Design review of the part shown in the three views and the two pictorial views. Dimensions are in mm from the part's minimum x, y and z. A direction names the side the tool comes from. Round coordinates to 2 decimals unless told otherwise and drop trailing zeros. Order: outer loops, then holes, each group sorted by start corner. A loop starts at its lowest first (then second) coordinate and runs counter-clockwise, first axis right, second up.
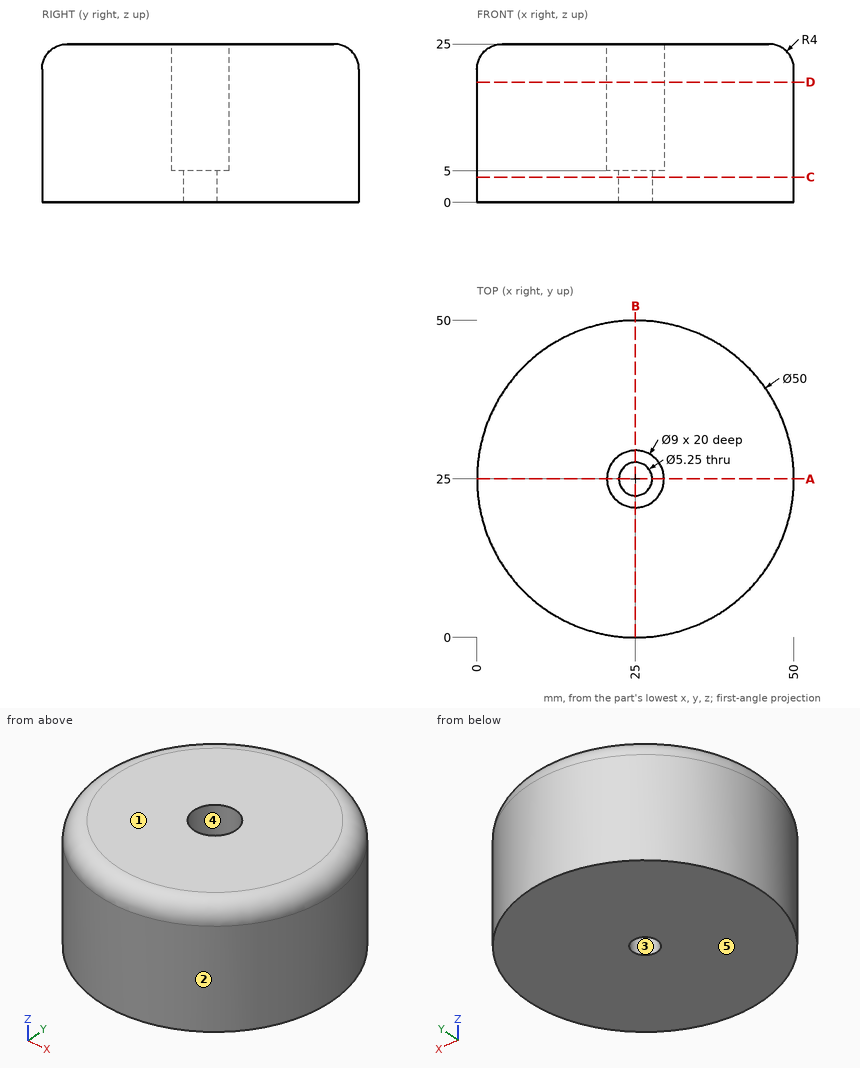
(1) Clearance check with flat-ended pins moving along their axes: P1, Ø1, axis at y = 32, z = 7.5, coming from the -X side; P2, Ø5, axis at y = 5, z = 12, coming from the -X side; P3, Ø11.5, axis at x = 25, y = 25, coming from the +Z side; P4, Ø4.5, axis at x = 24, y = 25, coming from the +Z side. State where each tip first meets the part, or that it passes through.
(2) Add section A-A on y = 25. Give the boundary of the cut face in (x, z) (3 decimals).
(3) Tool access review of the marked faces 4 and 5: name each direction out of +Z, -Z, +X, -X, +Y, -Y from which nothing blocks a thin tool from reaching the whole face with its end or side.
(4) Wall thickness on L1, parallel to Y at x = 25, z = 17.75; L2, parallel to Y at x = 25, z = 1.6 (3 decimals); L3, parallel to Y at x = 3, z = 7.25: over which ranges is each line inside the solid? List them lowest first.
(5) Add section D-D on z = 19. Give the boundary of the cut face in (x, y).
(6) Draft analysis for pull direction Y (two halves, no side actions). For the marked faces 1, 2 and 3, state which applies: pulls with the +Y half, pulls with the -Y half, needs draft (parallel to the pull), parting line crosses it, or undercut.
(7) Add section C-C on z = 4. Give the boundary of the cut face in (x, y) (3 decimals), plus the area to 3 significant figures.
Here are the results:
1. P1: stops at x = 0.86
1. P2: stops at x = 7.15
1. P3: stops at z = 25
1. P4: stops at z = 5
2. outline: (0, 0) - (22.375, 0) - (22.375, 5) - (20.5, 5) - (20.5, 25) - (4, 25) arc R4 ccw to (0, 21) - close; (27.625, 0) - (50, 0) - (50, 21) arc R4 ccw to (46, 25) - (29.5, 25) - (29.5, 5) - (27.625, 5) - close
3. face 4: +Z
3. face 5: -Z, +X, -X, +Y, -Y
4. L1: y = 0 to 20.5, 29.5 to 50
4. L2: y = 0 to 22.375, 27.625 to 50
4. L3: y = 13.13 to 36.87
5. outline: circle Ø50 at (25, 25); hole circle Ø9 at (25, 25)
6. face 1: needs draft
6. face 2: parting line crosses it
6. face 3: undercut
7. outline: circle Ø50 at (25, 25); hole circle Ø5.25 at (25, 25)
7. area: 1,940 mm2
